from build123d import *

# Parameters (mm, degrees)
SKETCH1_W           = 80
SKETCH1_H           = 180
SKETCH1_R           = 8.5
BOSS_EXTRUDE1_DEPTH = 5
SKETCH2_R           = 4.5
CUT_EXTRUDE1_DEPTH  = 30
SKETCH3_R           = 1.6
SKETCH3_R_2         = 2.5
CUT_EXTRUDE2_DEPTH  = 5
CUT_EXTRUDE3_DEPTH  = 10
BOSS_EXTRUDE2_DEPTH = 5
FILLET1_R           = 2
FILLET2_R           = 5
SKETCH6_R           = 2.1
CUT_EXTRUDE4_DEPTH  = 5
SKETCH7_W           = 60
SKETCH7_H           = 19.778044947
BOSS_EXTRUDE3_DEPTH = 5
SKETCH8_R           = 2.1
CUT_EXTRUDE6_DEPTH  = 5
CUT_EXTRUDE7_DEPTH  = 5
CUT_EXTRUDE8_DEPTH  = 10
FILLET3_R           = 5
FILLET4_R           = 3


with BuildPart() as part:
    # Sketch1 → Boss-Extrude1 (new body)
    with BuildSketch(Plane.XY):
        with Locations((10, 166)):
            Rectangle(SKETCH1_W, SKETCH1_H)
        with Locations((20, 226)):
            Circle(SKETCH1_R, mode=Mode.SUBTRACT)
    extrude(amount=BOSS_EXTRUDE1_DEPTH)

    # Sketch2 → Cut-Extrude1 (cut)
    with BuildSketch(Plane.XY.offset(5)):
        with Locations((20, 151)):
            Circle(SKETCH2_R)
    extrude(amount=-CUT_EXTRUDE1_DEPTH, mode=Mode.SUBTRACT)

    # Sketch3 → Cut-Extrude2 (cut)
    with BuildSketch(Plane.XY.offset(5)):
        with Locations((0, 182)):
            Circle(SKETCH3_R)
        with Locations((25, 129.301270189)):
            Circle(SKETCH3_R)
        with Locations((-25.032859693, 102.533479235)):
            Circle(SKETCH3_R)
        with Locations((-15, 81)):
            Circle(SKETCH3_R_2)
        with Locations((15, 81)):
            Circle(SKETCH3_R_2)
        with Locations((24, 91)):
            Circle(SKETCH3_R_2)
        with Locations((-24, 91)):
            Circle(SKETCH3_R_2)
    extrude(amount=-CUT_EXTRUDE2_DEPTH, mode=Mode.SUBTRACT)

    # Sketch4 → Cut-Extrude3 (cut)
    with BuildSketch(Plane.XY.offset(5)):
        with BuildLine():
            Line((-30, 194.384776311), (10.807611845, 235.192388155))
            ThreePointArc((10.807611845, 235.192388155), (24.974884621, 238.010433923), (33, 226))
            ThreePointArc((33, 226), (32.888783198, 224.303159501), (32.557035742, 222.635352414))
            Line((32.557035742, 222.635352414), (22.786943589, 186.172872106))
            Line((22.786943589, 186.172872106), (30, 173.679491924))
            Line((30, 173.679491924), (30, 76))
            Line((30, 76), (50, 76))
            Line((50, 76), (50, 256))
            Line((50, 256), (-30, 256))
            Line((-30, 256), (-30, 194.384776311))
        make_face()
    extrude(amount=-CUT_EXTRUDE3_DEPTH, mode=Mode.SUBTRACT)

    # Sketch5 → Boss-Extrude2 (add)
    with BuildSketch(Plane.XY.offset(5)):
        with BuildLine():
            Line((-30, 169.384776311), (-30, 194.384776311))
            Line((-30, 194.384776311), (-46.535533906, 177.849242405))
            ThreePointArc((-46.535533906, 177.849242405), (-47.619397663, 176.227125661), (-48, 174.313708499))
            Line((-48, 174.313708499), (-48, 96.071067812))
            ThreePointArc((-48, 96.071067812), (-47.619397663, 94.15765065), (-46.535533906, 92.535533906))
            Line((-46.535533906, 92.535533906), (-30, 76))
            Line((-30, 76), (-30, 101))
            ThreePointArc((-30, 101), (-35, 96), (-40, 101))
            Line((-40, 101), (-40, 131.707106781))
            Line((-40, 131.707106781), (-30, 121.707106781))
            Line((-30, 121.707106781), (-30, 138.67766953))
            Line((-30, 138.67766953), (-40, 148.67766953))
            Line((-40, 148.67766953), (-40, 169.384776311))
            ThreePointArc((-40, 169.384776311), (-35, 174.384776311), (-30, 169.384776311))
        make_face()
    extrude(amount=-BOSS_EXTRUDE2_DEPTH)

    # Fillet1
    fillet1_edges = [part.edges().sort_by_distance(p)[0] for p in [
        (-30, 121.707106781, 2.5),
        (-40, 131.707106781, 2.5),
        (-40, 148.67766953, 2.5),
        (-30, 138.67766953, 2.5),
    ]]
    fillet(fillet1_edges, radius=FILLET1_R)

    # Fillet2
    fillet2_edges = [part.edges().sort_by_distance(p)[0] for p in [
        (30, 173.679491924, 2.5),
        (22.786943589, 186.172872106, 2.5),
    ]]
    fillet(fillet2_edges, radius=FILLET2_R)

    # Sketch6 → Cut-Extrude4 (cut)
    with BuildSketch(Plane.XY.offset(5)):
        with Locations((15.982125076, 183.959163508)):
            Circle(SKETCH6_R)
    extrude(amount=-CUT_EXTRUDE4_DEPTH, mode=Mode.SUBTRACT)

    # Sketch7 → Boss-Extrude3 (add)
    with BuildSketch(Plane.XY.offset(5)):
        with Locations((0, 85.889022474)):
            Rectangle(SKETCH7_W, SKETCH7_H)
    extrude(amount=-BOSS_EXTRUDE3_DEPTH)

    # Sketch8 → Cut-Extrude6 (cut)
    with BuildSketch(Plane.XY.offset(5)):
        with Locations((-24, 81)):
            Circle(SKETCH8_R)
        with Locations((24, 81)):
            Circle(SKETCH8_R)
    extrude(amount=-CUT_EXTRUDE6_DEPTH, mode=Mode.SUBTRACT)

    # Sketch9 → Cut-Extrude7 (cut)
    with BuildSketch(Plane.XY.offset(5)):
        with BuildLine():
            Line((18.046029168, 201.838654795), (15.618513493, 192.779042959))
            ThreePointArc((15.618513493, 192.779042959), (13.91917225, 190.174254019), (11.008699323, 189.077972384))
            Line((11.008699323, 189.077972384), (-9.794056189, 188.162535924))
            ThreePointArc((-9.794056189, 188.162535924), (-14.590082182, 191.143181287), (-13.549405056, 196.693235631))
            Line((-13.549405056, 196.693235631), (1.27739155, 211.520032237))
            ThreePointArc((1.27739155, 211.520032237), (4.701786886, 212.983263), (8.18783091, 211.673673466))
            ThreePointArc((8.18783091, 211.673673466), (11.25, 209.430341871), (14.723866695, 207.900091446))
            ThreePointArc((14.723866695, 207.900091446), (17.601026512, 205.53588353), (18.046029168, 201.838654795))
        make_face()
    extrude(amount=-CUT_EXTRUDE7_DEPTH, mode=Mode.SUBTRACT)

    # Sketch10 → Cut-Extrude8 (cut)
    with BuildSketch(Plane.XY.offset(5)):
        Polygon((-20, 175.052757164), (-20, 110.591633523), (16.036879799, 175.052757164), align=None)
        with BuildLine():
            Line((12.329553187, 143.829627228), (-20, 86))
            Line((-20, 86), (18, 86))
            Line((18, 86), (18, 140.692235936))
            ThreePointArc((18, 140.692235936), (14.916675161, 141.812518921), (12.329553187, 143.829627228))
        make_face()
    extrude(amount=-CUT_EXTRUDE8_DEPTH, mode=Mode.SUBTRACT)

    # Fillet3
    fillet3_edges = [part.edges().sort_by_distance(p)[0] for p in [
        (18, 86, 2.5),
        (-20, 86, 2.5),
        (-20, 175.052757164, 2.5),
        (16.036879799, 175.052757164, 2.5),
        (-20, 110.591633523, 2.5),
    ]]
    fillet(fillet3_edges, radius=FILLET3_R)

    # Fillet4
    fillet4_edges = [part.edges().sort_by_distance(p)[0] for p in [
        (12.329553187, 143.829627228, 2.5),
        (18, 140.692235936, 2.5),
    ]]
    fillet(fillet4_edges, radius=FILLET4_R)


solid = part.part
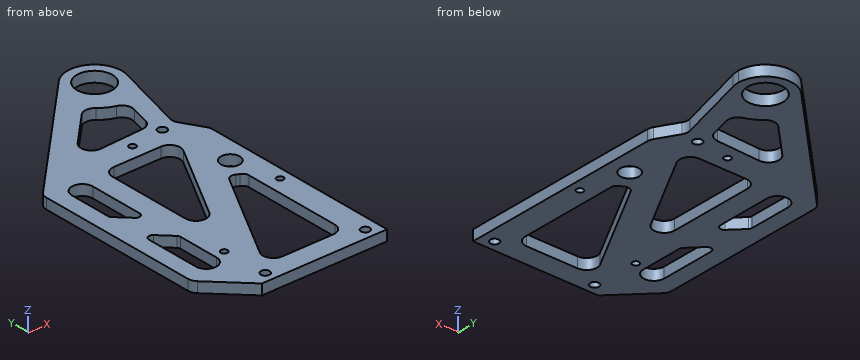
For this review, take the finished solid that the model builds, in its own axes (mm). Round coordinates to 2 decimals unless told otherwise and drop trailing zeros. Write each loop counter-clockwise with the first axis right and the second up, starting at its lowest first coordinate (ties: lowest second). Pieces come first, ordered by that corner, then holes. Notation, with made-up numbers: M -39,19.25 L -18,19.25 A25 cw -18,39.25 Z; hole C 5,-12 d3. An arc over 180 degrees is marked long. Write item = value, one per line. Start each with the question number.
(1) We need section C-C (z = 3.6). Give the number of separate pieces and of enclosed holes in the cut face, then the cut area to 3 significant figures.
(2) We need section D-D (y = 214.5). Give the boundary of the cut face in (x, z).
(3) We need section B-B (x = -35). Give the boundary of the cut face in (y, z).
(4) We need section A-A (y = 81). Give the boundary of the cut face in (x, z), then the cut area to 3 significant figures.
(5) For line 1 along X through (y, z) = (104.5, 2.15); line 2 along Y through (x, z) = (-4.5, 2.6); line 3 along Y through (x, z) = (-2, 1.1), list the stretches that pass through material, from the lowest coordinate up.
(6) Clearance check with flat-ended pins moving along their axes: pin 1 Ø2.5 at (y, z) = (115, 3.5) entering from +X; pin 2 Ø1.5 at (x, z) = (-3.5, 3) entering from +Y; pin 3 Ø3 at (y, z) = (190.5, 2.5) entering from -X. State where each tip first meets the part, or that it passes through.
Results found:
q1.separate_pieces = 1
q1.enclosed_holes = 13
q1.area = 6,660 mm²
q2.outline = M -9.88,0 L 30.38,0 L 30.38,5 L -9.88,5 Z
q3.outline = M 81,0 L 96,0 L 96,5 L 81,5 Z; M 126.71,0 L 143.68,0 L 143.68,5 L 126.71,5 Z; M 174.38,0 L 189.38,0 L 189.38,5 L 174.38,5 Z
q4.outline = M -35,0 L -26.1,0 L -26.1,5 L -35,5 Z; M -21.9,0 L 21.9,0 L 21.9,5 L -21.9,5 Z; M 26.1,0 L 30,0 L 30,5 L 26.1,5 Z
q4.area = 283 mm²
q5.line_1 = -48 to -40, -30 to -9.66, 18 to 30
q5.line_2 = 76 to 86, 113.73 to 138.32, 175.05 to 188.4, 205.74 to 219.88
q5.line_3 = 76 to 86, 118.2 to 142.79, 175.05 to 188.51, 208.24 to 222.38
q6.pin_1 = 30
q6.pin_2 = 221.63
q6.pin_3 = -35.38
